The model under review builds one solid part; all positions refer to its coordinate system, in mm. Round coordinates to 2 decimals unless told otherwise and drop trailing zeros. Order: outer loops, then holes, each group sorted by start corner. A loop starts at its lowest first (then second) coordinate and runs counter-clockwise, first axis right, second up.
from build123d import *

# Parameters (mm, degrees)
F0_R            = 2.5
F0_R_2          = 2.04
F1_DEPTH        = 1
F2_W            = 15
F2_H            = 15
F2_R            = 5
F2_R_2          = 2.5
F2_R_3          = 2.04
F3_DEPTH        = 1
F4_R            = 3
F5_R            = 0.75
F6_DEPTH        = 25
F6_COPIES_COUNT = 4


# Not quite as in the source:
# - a pattern or mirror of a feature is missing from the dataset's text; its kind, count and spacing are read off the source's solid


with BuildPart() as f1:
    # F0 (on Top) → F1 (new body)
    with BuildSketch(Plane.XY):
        Circle(F0_R)
        Circle(F0_R_2, mode=Mode.SUBTRACT)
    extrude(amount=F1_DEPTH)

    # F2 (on face) → F3 (join)
    with BuildSketch(Plane(origin=(0, 0, 0), x_dir=(1, 0, 0), z_dir=(0, 0, -1))):
        Rectangle(F2_W, F2_H)
        Circle(F2_R, mode=Mode.SUBTRACT)
        Circle(F2_R)
        Circle(F2_R_2, mode=Mode.SUBTRACT)
        Circle(F2_R_2)
        Circle(F2_R_3, mode=Mode.SUBTRACT)
    extrude(amount=F3_DEPTH)

    # F4
    f4_edges = [f1.edges().sort_by_distance(p)[0] for p in [
        (-7.5, 7.5, -0.5),
        (7.5, 7.5, -0.5),
        (-7.5, -7.5, -0.5),
        (7.5, -7.5, -0.5),
    ]]
    fillet(f4_edges, radius=F4_R)

    # F5 (on face) → F6 (cut)
    with BuildSketch(Plane.XY):
        with Locations((-4.5, 4.5)):
            Circle(F5_R)
        with Locations((-1.5, 4.5)):
            Circle(F5_R)
    f6 = extrude(amount=-F6_DEPTH, mode=Mode.SUBTRACT)

    # F6_copies: F6 ×4 about axis
    f6_copies_axis = Axis((0, 0, 0), (0, 0, 1))
    for i in range(1, F6_COPIES_COUNT):
        add(f6.rotate(f6_copies_axis, i * 360 / F6_COPIES_COUNT), mode=Mode.SUBTRACT)


solid = f1.part
(1) The part is to be moulded in two halves that separate along X. For faces 1 (the cylindrical face through (-4.044, -5.095, -0.493)), 2 (the cylindrical face through (5.095, -4.044, -0.493)), 3 (the flat face through (-2, -2, 0)), 4 (the cylindrical face through (-0.54, -2.44, 0.49)), say which applies: pulls with the +X half, pulls with the -X half, needs draft (parallel to the pull), parting line crosses it, or undercut.
(2) To check wall thickness, follow L1, parallel to X at y = -4.5, z = -0.45; L2, parallel to Y at x = -4.5, z = -0.2; L3, parallel to Y at x = -4, z = -0.8. State the ranges of each line that lie inside material, in increasing order.
(3) We need section A-A (x = 0). Give the boundary of the cut face in (y, z), and give its area (3 significant figures).
(4) We need section B-B (z = -0.5). Count the separate pieces of the cut face and the enclosed holes in it, and give its area (3 significant figures).
(5) We need section C-C (y = 4). Give the boundary of the cut face in (x, z), and give its area (3 significant figures).
(6) We need section D-D (x = -1.5). Give the boundary of the cut face in (y, z), and give its area (3 significant figures).
(7) Clearance check with flat-ended pins moving along their axes: P1, Ø1.2, axis at x = 1.5, y = -4.5, coming from the +Z side; P2, Ø1.5, axis at x = 4, y = 2.5, coming from the +Z side. State where each tip first meets the part, or that it passes through.
Verdict:
1. face 1: undercut
1. face 2: undercut
1. face 3: needs draft
1. face 4: parting line crosses it
2. L1: x = -7.5 to -5.25, -3.75 to 0.75, 2.25 to 3.75, 5.25 to 7.5
2. L2: y = -7.5 to -5.25, -3.75 to -2.25, -0.75 to 3.75, 5.25 to 7.5
2. L3: y = -7.5 to -5.06, -3.94 to -2.06, -0.94 to 3.94, 5.06 to 7.5
3. outline: (-7.5, -1) - (-2.04, -1) - (-2.04, 1) - (-2.5, 1) - (-2.5, 0) - (-7.5, 0) - close; (2.04, -1) - (7.5, -1) - (7.5, 0) - (2.5, 0) - (2.5, 1) - (2.04, 1) - close
3. area: 11.8 mm2
4. separate pieces: 1
4. enclosed holes: 9
4. area: 190 mm2
5. outline: (-7.5, -1) - (-5.06, -1) - (-5.06, 0) - (-7.5, 0) - close; (-3.94, -1) - (-2.06, -1) - (-2.06, 0) - (-3.94, 0) - close; (-0.94, -1) - (3.94, -1) - (3.94, 0) - (-0.94, 0) - close; (5.06, -1) - (7.5, -1) - (7.5, 0) - (5.06, 0) - close
5. area: 11.6 mm2
6. outline: (-7.5, -1) - (-1.38, -1) - (-1.38, 1) - (-2, 1) - (-2, 0) - (-7.5, 0) - close; (1.38, -1) - (3.75, -1) - (3.75, 0) - (2, 0) - (2, 1) - (1.38, 1) - close; (5.25, -1) - (7.5, -1) - (7.5, 0) - (5.25, 0) - close
6. area: 12.0 mm2
7. P1: passes through
7. P2: stops at z = 0
